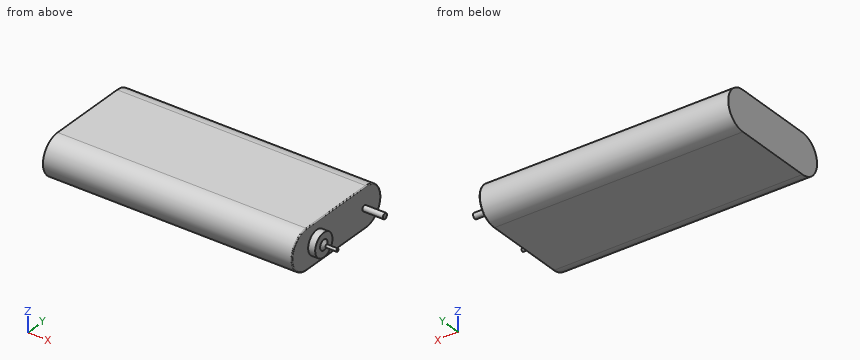
from build123d import *

# Parameters (mm, degrees)
BOSS_EXTRUDE1_DEPTH = 34.9885
SKETCH2_W           = 2.8956
SKETCH2_H           = 0.3937
FILLET1_R           = 0.127
CHAMFER1_SIZE       = 0.508
CHAMFER1_SIZE2      = 0.381


with BuildPart() as part:
    # Sketch1 → Boss-Extrude1 (new body)
    with BuildSketch(Plane(origin=(0, 0, 0), x_dir=(0, -1, 0), z_dir=(-1, 0, 0))):
        with BuildLine():
            Line((5.7023, 2.794), (-5.7023, 2.794))
            ThreePointArc((-5.7023, 2.794), (-8.4963, 0), (-5.7023, -2.794))
            Line((-5.7023, -2.794), (5.7023, -2.794))
            ThreePointArc((5.7023, -2.794), (8.4963, 0), (5.7023, 2.794))
        make_face()
    extrude(amount=-BOSS_EXTRUDE1_DEPTH)

    # Sketch2 → Revolve1 (revolve)
    with BuildSketch(Plane.XY, mode=Mode.PRIVATE) as revolve1_sk:
        with Locations((36.4363, 5.54355)):
            Rectangle(SKETCH2_W, SKETCH2_H)
    revolve(revolve1_sk.sketch.rotate(Axis((34.9885, 5.3467, 0), (1, 0, 0)), 270), axis=Axis((34.9885, 5.3467, 0), (1, 0, 0)))

    # Sketch3 → Revolve2 (revolve)
    with BuildSketch(Plane.XY, mode=Mode.PRIVATE) as revolve2_sk:
        Polygon((34.9885, -2.1082), (34.9885, -3.7592), (37.8841, -3.7592), (37.8841, -3.556), (35.9791, -3.556), (35.9791, -2.1082), align=None)
    revolve(revolve2_sk.sketch.rotate(Axis((34.9885, -3.7592, 0), (1, 0, 0)), 270), axis=Axis((34.9885, -3.7592, 0), (1, 0, 0)))

    # Fillet1
    fillet1_edges = [part.edges().sort_by_distance(p)[0] for p in [
        (34.9885, 8.4963, 0),
        (34.9885, 0, -2.794),
        (34.9885, -8.4963, 0),
        (34.9885, 0, 2.794),
    ]]
    fillet(fillet1_edges, radius=FILLET1_R)

    # Chamfer1
    chamfer1_edges = [part.edges().sort_by_distance(p)[0] for p in [
        (35.9791, -3.7592, 0.2032),
    ]]
    chamfer1_side = [part.faces().sort_by_distance(p)[0] for p in [
        (35.9791, -3.7592, 0.249897332),
    ]]
    chamfer(chamfer1_edges, length=CHAMFER1_SIZE, length2=CHAMFER1_SIZE2, reference=chamfer1_side[0])


solid = part.part
Input: part model. Units: mm. Frame: model coordinates. Coordinates: 2 decimals unless noted, no trailing zeros. Order: outer loops, then holes, each group sorted by start corner. A loop starts at its lowest first (then second) coordinate and runs counter-clockwise, first axis right, second up. Notation, with made-up numbers: M 17,30.5 L 51,30.5 A8 ccw 51,35.5 Z; hole C 19.5,-2 d10. An arc over 180 degrees is marked long. Write item = value, one per line. Start each with the question number.
(1) Section C-C on y = -2.5. Output: boundary loops of the cut face in (x, z).
(2) Section A-A on y = 1.75. Output: boundary loops of the cut face in (x, z).
(3) Section B-B on x = 16. Output: boundary loops of the cut face in (y, z).
(4) Line query: line 1 along X through (y, z) = (-1, -1.45); line 2 along X through (y, z) = (-3, -0.35); line 3 along Y through (x, z) = (5, -2.05). Output: solid intervals per line, ascending. Write a range as [from, to].
(5) First-contact query: P1, Ø1.5, axis at y = -2, z = -2, coming from the +X side. Flat tip, straight axial feed; report the tip coordinate or a pass-through.
Result set:
q1.outline = M 0,-2.79 L 34.86,-2.79 A0.13 ccw 34.99,-2.67 L 34.99,-1.07 L 35.98,-1.07 L 35.98,1.07 L 34.99,1.07 L 34.99,2.67 A0.13 ccw 34.86,2.79 L 0,2.79 Z
q2.outline = M 0,-2.79 L 34.86,-2.79 A0.13 ccw 34.99,-2.67 L 34.99,2.67 A0.13 ccw 34.86,2.79 L 0,2.79 Z
q3.outline = M -5.7,-2.79 L 5.7,-2.79 A2.79 ccw 5.7,2.79 L -5.7,2.79 A2.79 ccw Z
q4.line_1 = [0, 34.99]
q4.line_2 = [0, 35.98]
q4.line_3 = [-7.6, 7.6]
q5.P1 = 34.99
